from build123d import *

# Parameters (mm, degrees)
BOSS_EXTRU_1_DEPTH      = 5
ENL_V_MAT_EXTRU_1_DEPTH = 2
ESQUISSE7_R             = 6.5
ENL_V_MAT_EXTRU_3_DEPTH = 144.034294879
ESQUISSE10_R            = 3.175
ENL_V_MAT_EXTRU_4_DEPTH = 144.034294879
ESQUISSE11_W            = 6.6
ESQUISSE11_H            = 6.6
ENL_V_MAT_EXTRU_5_DEPTH = 3.5
BOSS_EXTRU_8_DEPTH      = 20
ESQUISSE18_W            = 70
ESQUISSE18_H            = 20
ESQUISSE18_W_2          = 62
ESQUISSE18_H_2          = 12
BOSS_EXTRU_9_DEPTH      = 30
ESQUISSE19_R            = 3.25
ENL_V_MAT_EXTRU_6_DEPTH = 140.679208812
ESQUISSE20_W            = 6.6
ESQUISSE20_H            = 6.6
ENL_V_MAT_EXTRU_7_DEPTH = 4
ESQUISSE21_W            = 40
ESQUISSE21_H            = 10
ENL_V_MAT_EXTRU_8_DEPTH = 147.060978744
ENL_V_MAT_EXTRU_9_DEPTH = 155.943014199


with BuildPart() as part:
    # Esquisse2 → Boss.-Extru.1 (new body)
    with BuildSketch(Plane(origin=(0, 0, 0), x_dir=(1, 0, 0), z_dir=(0, 1, 0))):
        with BuildLine():
            Line((79.497474683, -37.071067812), (42.426406871, 0))
            Line((42.426406871, 0), (79.497474683, 37.071067812))
            ThreePointArc((79.497474683, 37.071067812), (79.497474683, 79.497474683), (37.071067812, 79.497474683))
            Line((37.071067812, 79.497474683), (0, 42.426406871))
            Line((0, 42.426406871), (-37.071067812, 79.497474683))
            ThreePointArc((-37.071067812, 79.497474683), (-79.497474683, 79.497474683), (-79.497474683, 37.071067812))
            Line((-79.497474683, 37.071067812), (-42.426406871, 0))
            Line((-42.426406871, 0), (-79.497474683, -37.071067812))
            ThreePointArc((-79.497474683, -37.071067812), (-79.497474683, -79.497474683), (-37.071067812, -79.497474683))
            Line((-37.071067812, -79.497474683), (-30, -72.426406871))
            Line((-30, -72.426406871), (-30, -82.426406871))
            ThreePointArc((-30, -82.426406871), (0, -112.426406871), (30, -82.426406871))
            Line((30, -82.426406871), (30, -72.426406871))
            Line((30, -72.426406871), (37.071067812, -79.497474683))
            ThreePointArc((37.071067812, -79.497474683), (79.497474683, -79.497474683), (79.497474683, -37.071067812))
        make_face()
    extrude(amount=BOSS_EXTRU_1_DEPTH)

    # Esquisse4 → Enlèv. mat.-Extru.1 (cut)
    with BuildSketch(Plane(origin=(0, 0, 0), x_dir=(-1, 0, 0), z_dir=(0, -1, 0))):
        with BuildLine():
            Line((-33.535533906, -33.535533906), (-18.245921943, -18.245921943))
            Line((-18.245921943, -18.245921943), (-28.852523661, -7.639320225))
            Line((-28.852523661, -7.639320225), (-46.53019319, -25.316989755))
            ThreePointArc((-46.53019319, -25.316989755), (-39.575984314, -28.703872332), (-33.535533906, -33.535533906))
        make_face()
        with BuildLine():
            Line((-7.639320225, -28.852523661), (-18.245921943, -18.245921943))
            Line((-18.245921943, -18.245921943), (-33.535533906, -33.535533906))
            ThreePointArc((-33.535533906, -33.535533906), (-28.703872332, -39.575984314), (-25.316989755, -46.53019319))
            Line((-25.316989755, -46.53019319), (-7.639320225, -28.852523661))
        make_face()
        with BuildLine():
            ThreePointArc((-46.53019319, 25.316989755), (-33.535533906, 33.535533906), (-25.316989755, 46.53019319))
            Line((-25.316989755, 46.53019319), (-7.639320225, 28.852523661))
            Line((-7.639320225, 28.852523661), (-28.852523661, 7.639320225))
            Line((-28.852523661, 7.639320225), (-46.53019319, 25.316989755))
        make_face()
        with BuildLine():
            ThreePointArc((25.316989755, 46.53019319), (33.535533906, 33.535533906), (46.53019319, 25.316989755))
            Line((46.53019319, 25.316989755), (28.852523661, 7.639320225))
            Line((28.852523661, 7.639320225), (7.639320225, 28.852523661))
            Line((7.639320225, 28.852523661), (25.316989755, 46.53019319))
        make_face()
        with BuildLine():
            ThreePointArc((46.53019319, -25.316989755), (33.535533906, -33.535533906), (25.316989755, -46.53019319))
            Line((25.316989755, -46.53019319), (7.639320225, -28.852523661))
            Line((7.639320225, -28.852523661), (28.852523661, -7.639320225))
            Line((28.852523661, -7.639320225), (46.53019319, -25.316989755))
        make_face()
    extrude(amount=-ENL_V_MAT_EXTRU_1_DEPTH, mode=Mode.SUBTRACT)

    # Esquisse7 → Enlèv. mat.-Extru.3 (cut, through all)
    with BuildSketch(Plane(origin=(0, 0, 0), x_dir=(-1, 0, 0), z_dir=(0, -1, 0))):
        with Locations(Location((0, -82.426406871, 0), (0, 0, 90))):
            Circle(ESQUISSE7_R)
        with Locations(Location((-58.284271247, -58.284271247, 0), (0, 0, 90))):
            Circle(ESQUISSE7_R)
        with Locations(Location((-58.284271247, 58.284271247, 0), (0, 0, 90))):
            Circle(ESQUISSE7_R)
        with Locations(Location((58.284271247, 58.284271247, 0), (0, 0, 90))):
            Circle(ESQUISSE7_R)
        with Locations(Location((58.284271247, -58.284271247, 0), (0, 0, 90))):
            Circle(ESQUISSE7_R)
    extrude(amount=-ENL_V_MAT_EXTRU_3_DEPTH, mode=Mode.SUBTRACT)

    # Esquisse10 → Enlèv. mat.-Extru.4 (cut, through all)
    with BuildSketch(Plane(origin=(0, 5, 0), x_dir=(1, 0, 0), z_dir=(0, 1, 0))):
        with Locations(Location((25.403805922, -25.403805922, 0), (0, 0, 270))):
            Circle(ESQUISSE10_R)
        with Locations(Location((-25.403805922, -25.403805922, 0), (0, 0, 270))):
            Circle(ESQUISSE10_R)
        with Locations(Location((-25.403805922, 25.403805922, 0), (0, 0, 270))):
            Circle(ESQUISSE10_R)
        with Locations(Location((25.403805922, 25.403805922, 0), (0, 0, 270))):
            Circle(ESQUISSE10_R)
    extrude(amount=-ENL_V_MAT_EXTRU_4_DEPTH, mode=Mode.SUBTRACT)

    # Esquisse11 → Enlèv. mat.-Extru.5 (cut)
    with BuildSketch(Plane(origin=(0, 5, 0), x_dir=(1, 0, 0), z_dir=(0, 1, 0))):
        with Locations((-25.403805922, -25.403805922)):
            Rectangle(ESQUISSE11_W, ESQUISSE11_H)
        with Locations((25.403805922, -25.403805922)):
            Rectangle(ESQUISSE11_W, ESQUISSE11_H)
        with Locations((-25.403805922, 25.403805922)):
            Rectangle(ESQUISSE11_W, ESQUISSE11_H)
        with Locations((25.403805922, 25.403805922)):
            Rectangle(ESQUISSE11_W, ESQUISSE11_H)
    extrude(amount=-ENL_V_MAT_EXTRU_5_DEPTH, mode=Mode.SUBTRACT)

    # Esquisse16 → Boss.-Extru.8 (add)
    with BuildSketch(Plane(origin=(0, 5, 0), x_dir=(1, 0, 0), z_dir=(0, 1, 0))):
        Polygon((47.702116935, 85.698237446), (10.478031818, 48.474152329), (23.340408221, 35.611775926), (60.564493338, 72.835861043), align=None)
        Polygon((-23.340408221, 35.611775926), (-60.564493338, 72.835861043), (-47.702116935, 85.698237446), (-10.478031818, 48.474152329), align=None)
    extrude(amount=BOSS_EXTRU_8_DEPTH)

    # Esquisse18 → Boss.-Extru.9 (add)
    with BuildSketch(Plane(origin=(0, 5, 0), x_dir=(1, 0, 0), z_dir=(0, 1, 0))):
        Rectangle(ESQUISSE18_W, ESQUISSE18_H)
        Rectangle(ESQUISSE18_W_2, ESQUISSE18_H_2, mode=Mode.SUBTRACT)
    extrude(amount=BOSS_EXTRU_9_DEPTH)

    # Esquisse19 → Enlèv. mat.-Extru.6 (cut, through all)
    with BuildSketch(Plane.XY.offset(10)):
        with Locations((0, 29)):
            Circle(ESQUISSE19_R)
    extrude(amount=-ENL_V_MAT_EXTRU_6_DEPTH, mode=Mode.SUBTRACT)

    # Esquisse20 → Enlèv. mat.-Extru.7 (cut)
    with BuildSketch(Plane.XY.offset(10)):
        with Locations((0, 29)):
            Rectangle(ESQUISSE20_W, ESQUISSE20_H)
    extrude(amount=-ENL_V_MAT_EXTRU_7_DEPTH, mode=Mode.SUBTRACT)

    # Esquisse21 → Enlèv. mat.-Extru.8 (cut, through all)
    with BuildSketch(Plane(origin=(0, 5, 0), x_dir=(1, 0, 0), z_dir=(0, 1, 0))):
        Rectangle(ESQUISSE21_W, ESQUISSE21_H)
    extrude(amount=-ENL_V_MAT_EXTRU_8_DEPTH, mode=Mode.SUBTRACT)

    # Esquisse22 → Enlèv. mat.-Extru.9 (cut, through all)
    with BuildSketch(Plane(origin=(0, 0, -10), x_dir=(-1, 0, 0), z_dir=(0, 0, -1))):
        Polygon((-10, 10), (10, 10), (0, 20), align=None)
    extrude(amount=-ENL_V_MAT_EXTRU_9_DEPTH, mode=Mode.SUBTRACT)


solid = part.part
The listing builds one solid part. Answer for the finished solid, in the listing's coordinates (mm). A direction names the side the tool comes from. Coordinates: 2 decimals unless noted, no trailing zeros. Write each loop counter-clockwise with the first axis right and the second up, starting at its lowest first coordinate (ties: lowest second). Pieces come first, ordered by that corner, then holes. Notation, with made-up numbers: M -18,70 L 32,70 A14 ccw 32,90 Z; hole C 51.5,87 d1. An arc over 180 degrees is marked long. Put each result on its own line as item: value. Start each with the question number.
1. A cutting plane is placed at A-A on y = 17. Write down the section's boundary in (x, z), then the cut area to 3 significant figures.
2. A cutting plane is placed at D-D on z = -17. Write down the section's boundary in (x, y), then the cut area to 3 significant figures.
3. Flat-ended cylindrical pins translate along their axes: P1, Ø25, axis at x = -43, z = -65, coming from the +Y side; P2, Ø17, axis at x = -58.28, z = -58.28, coming from the -Y side; P3, Ø10, axis at y = 19, z = -0.5, coming from the -X side; P4, Ø3.5, axis at x = -24, y = 4, coming from the -Z side. Find the tip coordinate at first contact, or state that the pin passes through.
4. For a pull along Z with two mould halves and no side action, classify faces 1 (the flat face through (-54.2, 14.9, -79.2)), 2 (the flat face through (-61.221, 2.465, -18.795)), 3 (the flat face through (-35, 25, -61)) as pulls with the +Z half, pulls with the -Z half, needs draft (parallel to the pull), parting line crosses it, or undercut.
5. Which of the six approach directions +Z, -Z, +X, -X, +Y, -Y give full straight-line access (tool end or side, diameter ignored) to faces 4 (the flat face through (31, 20, 0)), 5 (the flat face through (18.1, 0.99, 18.39)), 6 (the flat face through (-0.5, 19.8, -10)), 7 (the flat face through (54.2, 14.9, -79.2))?
6. A cutting plane is placed at B-B on y = 29. Write down the section's boundary in (x, z), then the cut area to 3 significant figures.
7. A cutting plane is placed at C-C on x = -15.5. Write down the section's boundary in (y, z), then the cut area to 3 significant figures.
8. Consider line 1 (Y direction, x = 0, z = -8); line 2 (X direction, y = 25, z = -5); line 3 (Z direction, x = 1.5, y = 20). Determine where each line is inside the solid, lowest interval first. Write a range as from..to.
Resolved:
1. outline: M -60.56,-72.84 L -47.7,-85.7 L -10.48,-48.47 L -23.34,-35.61 Z; M -35,-10 L -3,-10 L -3,-6 L -31,-6 L -31,6 L -3,6 L -3,10 L -35,10 Z; M 3,-10 L 35,-10 L 35,10 L 3,10 L 3,6 L 31,6 L 31,-6 L 3,-6 Z; M 10.48,-48.47 L 47.7,-85.7 L 60.56,-72.84 L 23.34,-35.61 Z
1. area: 2,520 mm2
2. outline: M -59.43,0 L -38.21,0 L -38.21,2 L -19.49,2 L -19.49,0 L 19.49,0 L 19.49,2 L 38.21,2 L 38.21,0 L 59.43,0 L 59.43,5 L -59.43,5 Z
2. area: 519 mm2
3. P1: stops at y = 25
3. P2: stops at y = 0
3. P3: stops at x = -35
3. P4: stops at z = -68.18
4. face 1: pulls with the -Z half
4. face 2: undercut
4. face 3: needs draft
5. face 4: +Y
5. face 5: -Y
5. face 6: +X, -X, +Y
5. face 7: -Z, +X, +Y
6. outline: M -35,-10 L -3.25,-10 L -3.25,-6 L -31,-6 L -31,6 L -3.3,6 L -3.3,10 L -35,10 Z; M 3.25,-10 L 35,-10 L 35,10 L 3.3,10 L 3.3,6 L 31,6 L 31,-6 L 3.25,-6 Z
6. area: 604 mm2
7. outline: M 0,-57.93 L 5,-57.93 L 5,-53.5 L 25,-53.5 L 25,-43.45 L 5,-43.45 L 5,-10 L 35,-10 L 35,-6 L 5,-6 L 5,-5 L 0,-5 L 0,-20.99 L 2,-20.99 L 2,-36.71 L 0,-36.71 Z; M 0,5 L 5,5 L 5,6 L 35,6 L 35,10 L 5,10 L 5,108.11 L 0,108.11 L 0,36.71 L 2,36.71 L 2,20.99 L 0,20.99 Z
7. area: 1,160 mm2
8. line 1: y = 0..10, 20..25.75, 32.25..35
8. line 2: x = -35..-31, 31..35
8. line 3: z = -10..-6, 6..10
